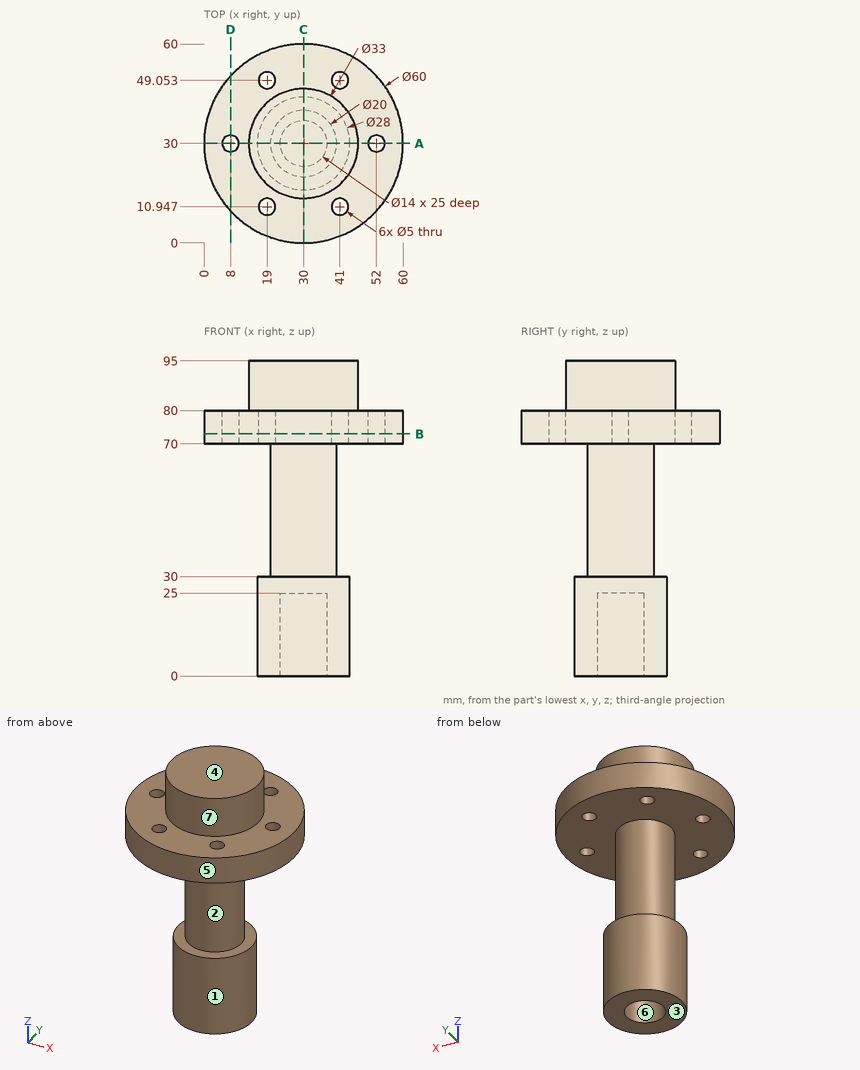
Verification items for this drawing (mm, ordinates from the low corner). A direction names the side the tool comes from. Coordinates: 2 decimals unless noted, no trailing zeros. Loops run counter-clockwise (first coordinate to the right, second up) from the corner with the lowest first, then second, coordinate; pieces in that order, holes last.
Item 1: Sectioned sample at C-C, the plane x = 30. Record the boundary of the cut face in (y, z).
Item 2: Access from +Z, -Z, +X, -X, +Y, -Y to the whole of each face (thin tool, end or side, straight path). Record for the marked faces 5, 6 and 7.
Item 3: Sectioned sample at A-A, the plane y = 30. Record the boundary of the cut face in (x, z), then the cut area to 4 significant figures.
Item 4: Go/stop test with flat-tipped pins: pin 1 Ø11 at (x, y) = (30.5, 29) entering from -Z; pin 2 Ø8 at (x, y) = (52, 30) entering from -Z; pin 3 Ø1 at (x, z) = (14, 72.5) entering from -Y (1 decimal); pin 4 Ø4 at (x, y) = (41, 49.05) entering from -Z. Record where each tip stops, or that it passes through.
Item 5: Release check for a two-part mould opening along Z. For the marked faces 1, 2, 3 and 4 record: released by +Z, released by -Z, zero draft, split by the parting line, or undercut.
Item 6: Sectioned sample at D-D, the plane x = 8. Record the boundary of the cut face in (y, z).
Item 7: Sectioned sample at B-B, the plane z = 73. Record the boundary of the cut face in (x, y).
Item 8: Thickness scan on line 1 (Y direction, x = 19, z = 73.25); line 2 (X direction, y = 11, z = 79) (1 decimal); line 3 (Z direction, x = 5, y = 36.5). Record the ranges inside material, lowest first.
Check result:
1. outline: (0, 70) - (20, 70) - (20, 30) - (16, 30) - (16, 0) - (23, 0) - (23, 25) - (37, 25) - (37, 0) - (44, 0) - (44, 30) - (40, 30) - (40, 70) - (60, 70) - (60, 80) - (46.5, 80) - (46.5, 95) - (13.5, 95) - (13.5, 80) - (0, 80) - close
2. face 5: +Z, -Z
2. face 6: -Z
2. face 7: +Z
3. outline: (0, 70) - (5.5, 70) - (5.5, 80) - (0, 80) - close; (10.5, 70) - (20, 70) - (20, 30) - (16, 30) - (16, 0) - (23, 0) - (23, 25) - (37, 25) - (37, 0) - (44, 0) - (44, 30) - (40, 30) - (40, 70) - (49.5, 70) - (49.5, 80) - (46.5, 80) - (46.5, 95) - (13.5, 95) - (13.5, 80) - (10.5, 80) - close; (54.5, 70) - (60, 70) - (60, 80) - (54.5, 80) - close
3. area: 2,285 mm2
4. pin 1: stops at z = 25
4. pin 2: stops at z = 70
4. pin 3: stops at y = 4.3
4. pin 4: passes through
5. face 1: zero draft
5. face 2: undercut
5. face 3: released by -Z
5. face 4: released by +Z
6. outline: (9.6, 70) - (27.5, 70) - (27.5, 80) - (9.6, 80) - close; (32.5, 70) - (50.4, 70) - (50.4, 80) - (32.5, 80) - close
7. outline: circle Ø60 at (30, 30); hole circle Ø5 at (8, 30); hole circle Ø5 at (19, 10.95); hole circle Ø5 at (19, 49.05); hole circle Ø5 at (41, 10.95); hole circle Ø5 at (41, 49.05); hole circle Ø5 at (52, 30)
8. line 1: y = 2.09 to 8.45, 13.45 to 46.55, 51.55 to 57.91
8. line 2: x = 6.8 to 16.5, 21.5 to 38.5, 43.5 to 53.2
8. line 3: z = 70 to 80
